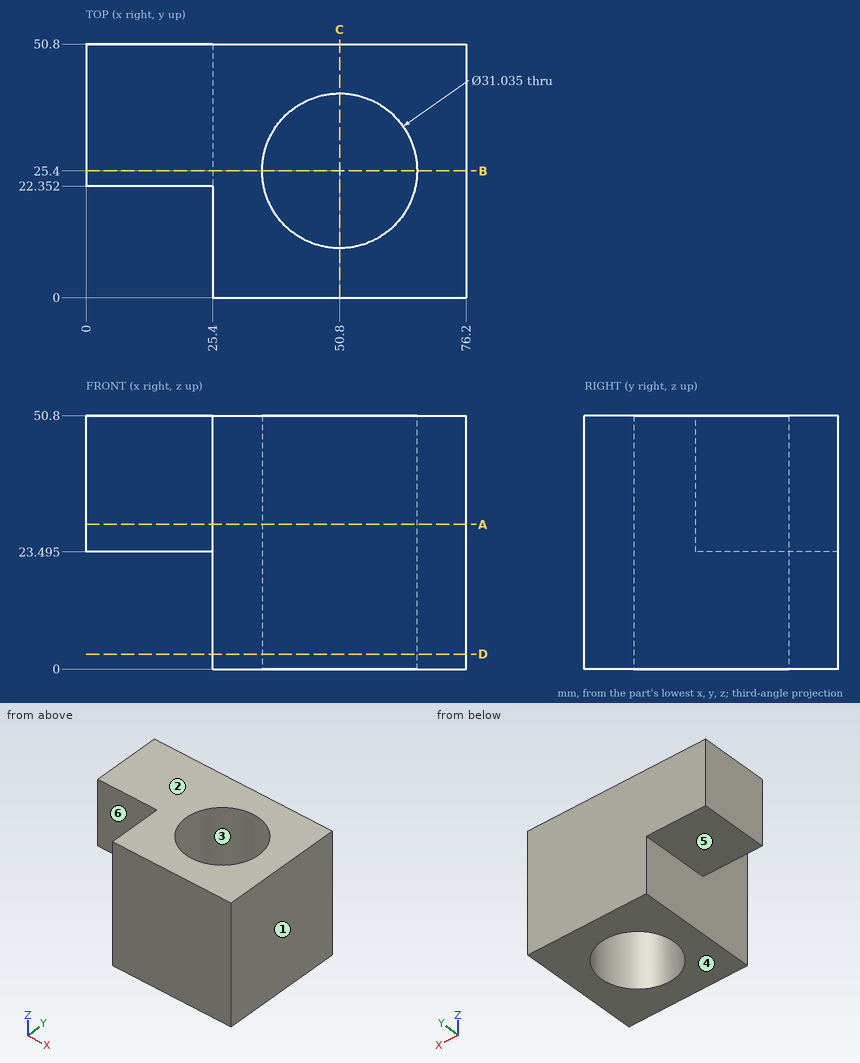
Job drawing, mm, ordinate dimensions from the low corner. One solid piece. A direction names the side the tool comes from. Give positions to 0.01 mm unless a question says otherwise; leave off trailing zeros. Order: outer loops, then holes, each group sorted by start corner. A loop starts at its lowest first (then second) coordinate and runs counter-clockwise, first axis right, second up. Notation, with made-up numbers: (40.25, -29) - (86.25, -29) arc R15 cw to (86.25, -7) - close; hole circle Ø9 at (6, 26.5). An arc over 180 degrees is marked (long way). Answer in a Markdown table with one row per item.
1. Probe probe 1 along Y at (x, z) = (50, 16); probe 2 along X at (y, z) = (25.4, 17); probe 3 along X at (y, z) = (25.4, 41). List the from-to ranges inside material, lowest first. Write a range as [from, to].
Data:
| item | result |
|---|---|
| probe 1 | y = [0, 9.9], [40.9, 50.8] |
| probe 2 | x = [25.4, 35.28], [66.32, 76.2] |
| probe 3 | x = [0, 35.28], [66.32, 76.2] |
2. Saw through at A-A, the plane z = 29. Give the cut face in (x, y) (1 decimal).
Data:
| item | result |
|---|---|
| outline | (0, 22.4) - (25.4, 22.4) - (25.4, 0) - (76.2, 0) - (76.2, 50.8) - (0, 50.8) - close; hole circle Ø31 at (50.8, 25.4) |
3. Saw through at B-B, the plane y = 25.4. Give the cut face in (x, z) (1 decimal), plus the area to 3 significant figures.
Data:
| item | result |
|---|---|
| outline | (0, 23.5) - (25.4, 23.5) - (25.4, 0) - (35.3, 0) - (35.3, 50.8) - (0, 50.8) - close; (66.3, 0) - (76.2, 0) - (76.2, 50.8) - (66.3, 50.8) - close |
| area | 1,700 mm² |
4. Tool access for the marked faces 4, 5 and 6: list every direction of +Z, -Z, +X, -X, +Y, -Y with a clear straight run to the whole face (end or side of a thin tool).
Data:
| item | result |
|---|---|
| face 4 | -Z, +X, -X, +Y, -Y |
| face 5 | -Z, -X, +Y, -Y |
| face 6 | +Z, -Z, -X, -Y |
5. Pull direction X, two halves, no side cores. Call the marked faces 1, 2 and 3: pulls with the +X half, pulls with the -X half, needs draft (parallel to the pull), parting line crosses it, or undercut.
Data:
| item | result |
|---|---|
| face 1 | pulls with the +X half |
| face 2 | needs draft |
| face 3 | undercut |
6. Saw through at D-D, the plane z = 3. Give the cut face in (x, y) (1 decimal).
Data:
| item | result |
|---|---|
| outline | (25.4, 0) - (76.2, 0) - (76.2, 50.8) - (25.4, 50.8) - close; hole circle Ø31 at (50.8, 25.4) |
7. Flat gauge pins, fed straight in: pin 1 (4 mm diameter, centred on y = 7.5, z = 18, fed in from -X); pin 2 (7.5 mm diameter, centred on x = 16, z = 37.5, fed in from -Y); pin 3 (7.5 mm diameter, centred on x = 9, y = 39, fed in from -Z) (3 decimals). Where does each tip first touch, or does it go through?
Data:
| item | result |
|---|---|
| pin 1 | stops at x = 25.4 |
| pin 2 | stops at y = 22.35 |
| pin 3 | stops at z = 23.495 |
8. Saw through at C-C, the plane x = 50.8. Give the cut face in (y, z), plus the area to 3 significant figures.
Data:
| item | result |
|---|---|
| outline | (0, 0) - (9.88, 0) - (9.88, 50.8) - (0, 50.8) - close; (40.92, 0) - (50.8, 0) - (50.8, 50.8) - (40.92, 50.8) - close |
| area | 1,000 mm² |
